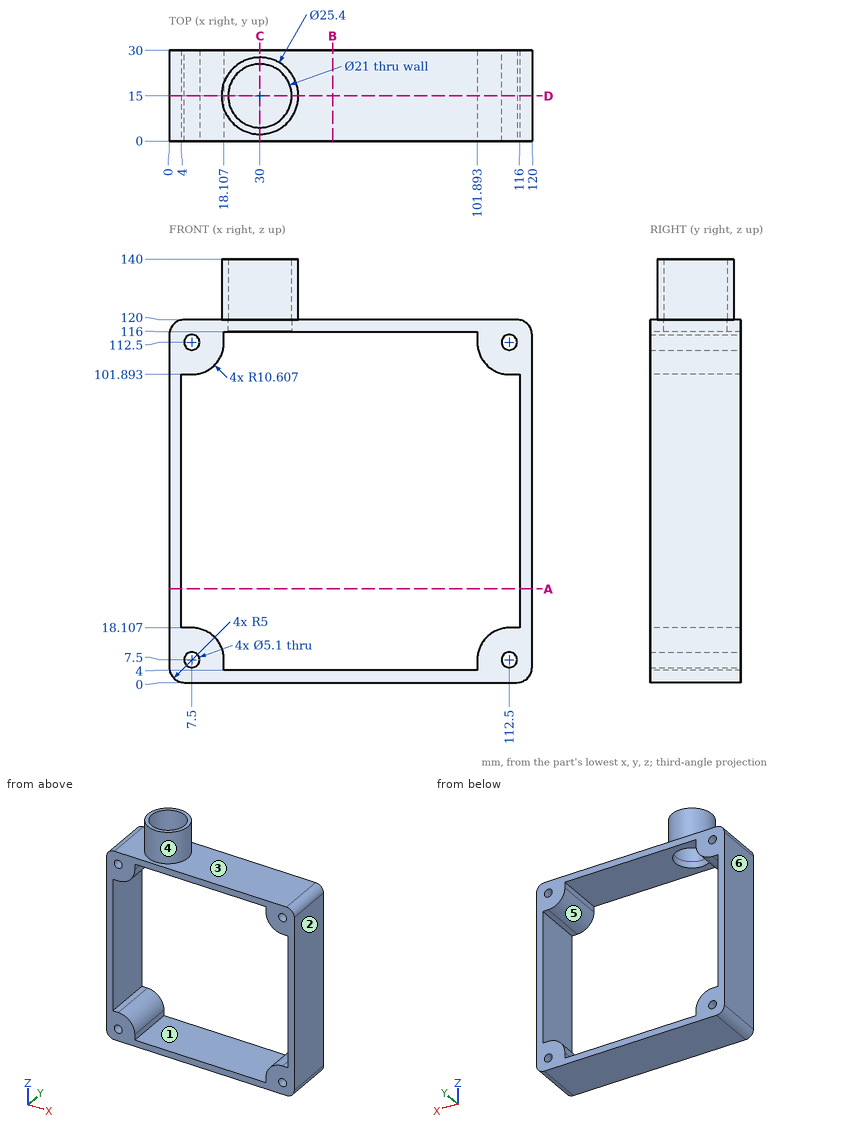
Part print with two shaded views. Sizes in mm from the minimum x, y, z corner. A direction names the side the tool comes from. Round coordinates to 2 decimals unless told otherwise and drop trailing zeros. Loops run counter-clockwise (first coordinate to the right, second up) from the corner with the lowest first, then second, coordinate; pieces in that order, holes last.
Item 1: Two-plate mould, pull along X, no slides. Class the marked faces 1, 2 and 3: released by +X, released by -X, zero draft, split by the parting line, or undercut.
Item 2: Drill centre lines: line 1 along Z through (x, y) = (112.5, 19.5); line 2 along Z through (x, y) = (55, 16.25); line 3 along X through (y, z) = (4.5, 113). Where is each one in solid material? Low to high.
Item 3: Pin check, flat tips, straight feed: P1, Ø3, axis at y = 22, z = 123, coming from the +X side; P2, Ø6, axis at x = 24, y = 11.5, coming from the +Z side; P3, Ø5, axis at x = 77.5, y = 25, coming from the +Z side; P4, Ø10, axis at x = 13.5, y = 18, coming from the +Z side. Stop position of each tip, or through.
Item 4: Which spindle directions (+Z, -Z, +X, -X, +Y, -Y) get a long thin tool onto all of the face, cutting with end or side? Do the marked faces 4, 5 and 6. Say none if no direction does.
Item 5: Saw through at B-B (x = 54). List the corners of the cut face in (y, z), then the cut area to 3 significant figures.
Item 6: Saw through at D-D (y = 15). State how many separate pieces and enclosed holes the cut face has, then the cut area to 3 significant figures.
Item 7: Saw through at C-C (x = 30). List the corners of the cut face in (y, z), then the cut area to 3 significant figures.
Item 8: Saw through at A-A (z = 31). List the corners of the cut face in (x, y).
Worked answers:
1. face 1: undercut
1. face 2: released by +X
1. face 3: zero draft
2. line 1: z = 0 to 4.95, 10.05 to 18.11, 101.89 to 109.95, 115.05 to 120
2. line 2: z = 0 to 4, 116 to 120
2. line 3: x = 0 to 5, 10 to 18.11, 101.89 to 110, 115 to 120
3. P1: stops at x = 41.45
3. P2: stops at z = 4
3. P3: stops at z = 120
3. P4: stops at z = 140
4. face 4: +Z
4. face 5: +Y, -Y
4. face 6: +Z, -Z, -X, +Y, -Y
5. outline: (0, 0) - (30, 0) - (30, 4) - (0, 4) - close; (0, 116) - (30, 116) - (30, 120) - (0, 120) - close
5. area: 240 mm2
6. separate pieces: 1
6. enclosed holes: 4
6. area: 2,460 mm2
7. outline: (0, 0) - (30, 0) - (30, 4) - (0, 4) - close; (0, 116) - (4.5, 116) - (4.5, 140) - (2.3, 140) - (2.3, 120) - (0, 120) - close; (25.5, 116) - (30, 116) - (30, 120) - (27.7, 120) - (27.7, 140) - (25.5, 140) - close
7. area: 244 mm2
8. outline: (0, 0) - (4, 0) - (4, 30) - (0, 30) - close; (116, 0) - (120, 0) - (120, 30) - (116, 30) - close
